Answer from the drawing. Dimensions are ordinates in mm from the lowest x, y and z of the part. Round coordinates to 2 decimals unless told otherwise and drop trailing zeros. Order: outer loops, then holes, each group sorted by start corner. A loop starts at its lowest first (then second) coordinate and runs counter-clockwise, first axis right, second up. Notation, with made-up numbers: (-3.5, -13.75) - (46.5, -13.75) arc R20 cw to (46.5, 13.25) - close; hole circle Ø11 at (77.25, 35.25). An arc over 180 degrees is marked (long way). One line per question, with ' | ' between items. Start each with the question number.
1) Flat-ended cylindrical pins translate along their axes: pin 1 (2.5 mm diameter, centred on x = 150.5, y = 3, fed in from +Z); pin 2 (4.5 mm diameter, centred on x = 79, z = 105, fed in from -Y); pin 3 (3 mm diameter, centred on x = 159.5, y = 4.5, fed in from -Z); pin 4 (1 mm diameter, centred on y = 1.5, z = 137, fed in from -X). Find the tip coordinate at first contact, or state that the pin passes through.
2) The part is cut by section B-B, the plane x = 79. Give the vertices of the cut face in (y, z).
3) The part is cut by section D-D, the plane z = 105. Give the vertices of the cut face in (x, y), plus the area to 3 significant figures.
4) The part is cut by section C-C, the plane x = 105. Give the vertices of the cut face in (y, z), plus the area to 3 significant figures.
5) Straight lines are drawn through the part: line 1 (Z direction, x = 105, y = 3.25); line 2 (X direction, y = 4.5, z = 140). For each, find the intervals that lie inside material, in ascending order. Write a range as from..to.
6) The part is cut by section A-A, the plane z = 79. Give the vertices of the cut face in (x, y), plus the area to 3 significant figures.
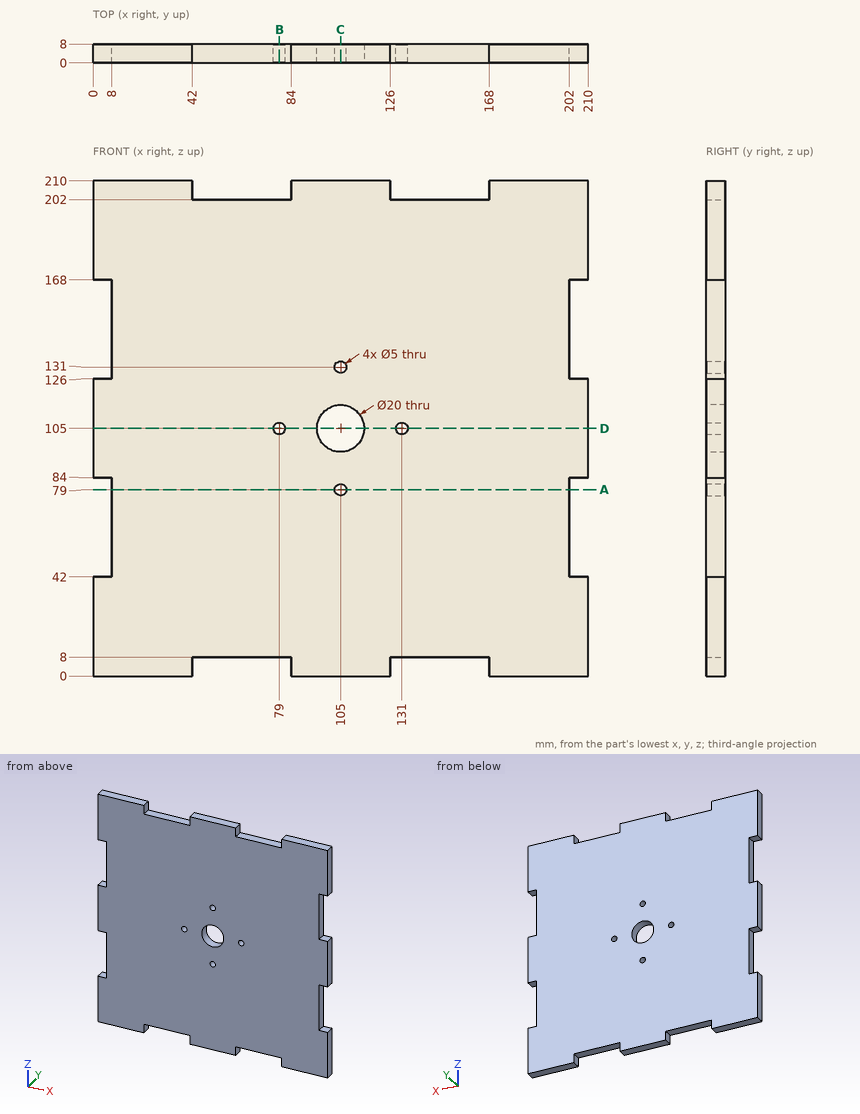
Values:
1) pin 1: stops at z = 202 | pin 2: passes through | pin 3: stops at z = 8 | pin 4: stops at x = 8
2) outline: (0, 8) - (8, 8) - (8, 102.5) - (0, 102.5) - close; (0, 107.5) - (8, 107.5) - (8, 202) - (0, 202) - close
3) outline: (0, 0) - (76.5, 0) - (76.5, 8) - (0, 8) - close; (81.5, 0) - (95, 0) - (95, 8) - (81.5, 8) - close; (115, 0) - (128.5, 0) - (128.5, 8) - (115, 8) - close; (133.5, 0) - (210, 0) - (210, 8) - (133.5, 8) - close | area: 1,440 mm^2
4) outline: (0, 0) - (8, 0) - (8, 76.5) - (0, 76.5) - close; (0, 81.5) - (8, 81.5) - (8, 95) - (0, 95) - close; (0, 115) - (8, 115) - (8, 128.5) - (0, 128.5) - close; (0, 133.5) - (8, 133.5) - (8, 210) - (0, 210) - close | area: 1,440 mm^2
5) line 1: z = 0..76.5, 81.5..95, 115..128.5, 133.5..210 | line 2: x = 8..202
6) outline: (8, 0) - (102.5, 0) - (102.5, 8) - (8, 8) - close; (107.5, 0) - (202, 0) - (202, 8) - (107.5, 8) - close | area: 1,510 mm^2
